Print and shaded views of the part. All mm, measured from the part's lowest x, y and z. A direction names the side the tool comes from. Round coordinates to 2 decimals unless told otherwise and drop trailing zeros. Write each loop counter-clockwise with the first axis right and the second up, starting at its lowest first coordinate (ties: lowest second). Pieces come first, ordered by that corner, then holes. Notation, with made-up numbers: (19, 81.25) -> (66, 81.25) arc R28 cw to (66, 100.25) -> close; hole circle Ø7 at (49, 18). An arc over 180 degrees is marked (long way). Return JSON: item names as keys, results as strings. Group by question number.
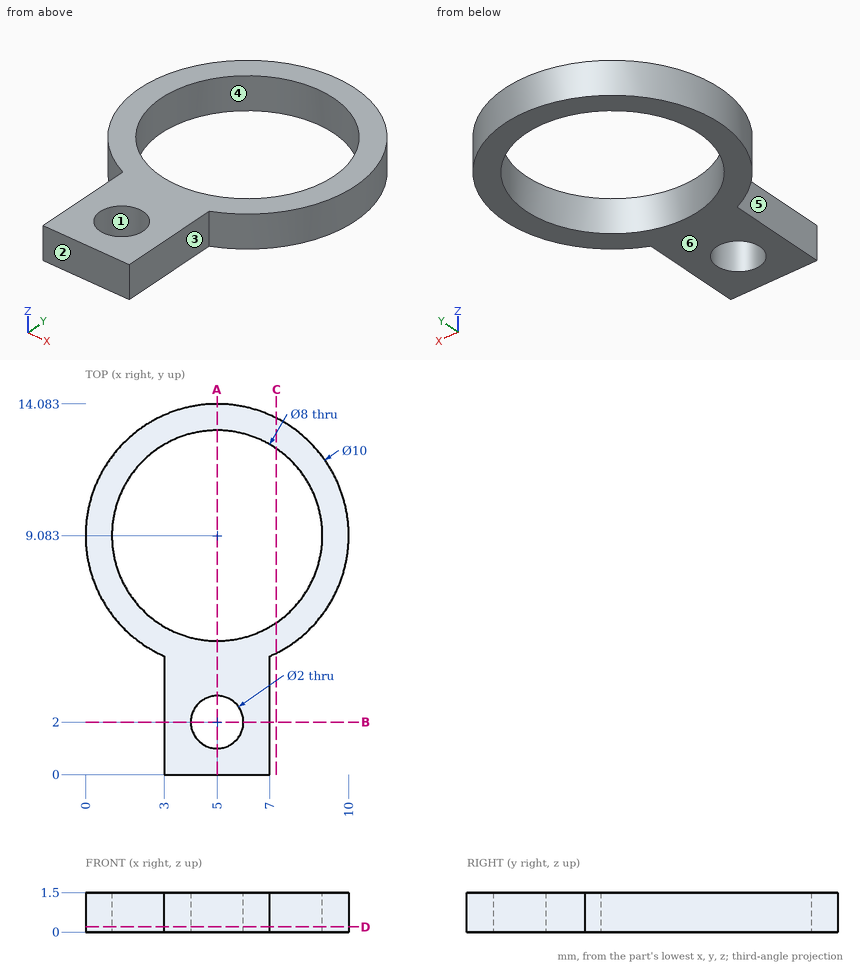
Item 1: Flat gauge pin, fed straight in: P1, Ø1.5, axis at x = 7.5, y = 10.5, coming from the +Z side. Where does the tip first touch, or does it go through?
Item 2: Two-plate mould, pull along Y, no slides. Class the marked faces 1, 2, 3 and 4: released by +Y, released by -Y, zero draft, split by the parting line, or undercut.
Item 3: Cut at A-A (x = 5). Write the cut outline in (y, z).
Item 4: Wall check: L1, parallel to Y at x = 5, z = 1; L2, parallel to X at y = 4, z = 0.2; L3, parallel to Y at x = 3.25, z = 0.55 (1 decimal). Give the ranges that are in metal, low to high.
Item 5: Cut at C-C (x = 7.25). Write the cut outline in (y, z) (1 decimal).
Item 6: Which spindle directions (+Z, -Z, +X, -X, +Y, -Y) get a long thin tool onto all of the face, cutting with end or side? Do the marked faces 5 and 6. Say none if no direction does.
Item 7: Cut at D-D (z = 0.2). Write the cut outline in (x, y).
Item 8: Cut at B-B (y = 2). Write the cut outline in (x, z).
Checks:
{
 "1": {"P1": "passes through"},
 "2": {"face 1": "undercut", "face 2": "released by -Y", "face 3": "zero draft", "face 4": "undercut"},
 "3": {"outline": "(0, 0) -> (1, 0) -> (1, 1.5) -> (0, 1.5) -> close; (3, 0) -> (5.08, 0) -> (5.08, 1.5) -> (3, 1.5) -> close; (13.08, 0) -> (14.08, 0) -> (14.08, 1.5) -> (13.08, 1.5) -> close"},
 "4": {"L1": "y = 0 to 1, 3 to 5.08, 13.08 to 14.08", "L2": "x = 3 to 7", "L3": "y = 0 to 5.5, 12.7 to 13.8"},
 "5": {"outline": "(4.6, 0) -> (5.8, 0) -> (5.8, 1.5) -> (4.6, 1.5) -> close; (12.4, 0) -> (13.5, 0) -> (13.5, 1.5) -> (12.4, 1.5) -> close"},
 "6": {"face 5": "+Z, -Z, -X, -Y", "face 6": "-Z, +X, -X, +Y, -Y"},
 "7": {"outline": "(3, 0) -> (7, 0) -> (7, 4.5) arc R5 ccw (long way) to (3, 4.5) -> close; hole circle Ø8 at (5, 9.08); hole circle Ø2 at (5, 2)"},
 "8": {"outline": "(3, 0) -> (4, 0) -> (4, 1.5) -> (3, 1.5) -> close; (6, 0) -> (7, 0) -> (7, 1.5) -> (6, 1.5) -> close"}
}
